from build123d import *

# Parameters (mm, degrees)
F1_DEPTH = 10
F2_DEPTH = 39
F3_R     = 1.27
F4_DEPTH = 39
F0_R     = 1.27
F5_DEPTH = 37


# Not quite as in the source:
# - a feature names something its author has since deleted; it is built from what else it names


with BuildPart() as f1:
    # F0 (on Top) → F1 (new body)
    with BuildSketch(Plane.XY):
        with BuildLine():
            Line((39.0916730868, 1.5), (-39.2084973779, 1.5))
            ThreePointArc((-39.2084973779, 1.5), (-39.0523737086, 0.7572105316), (-39, 0))
            ThreePointArc((-39, 0), (-39.0523737086, -0.7572105316), (-39.2084973779, -1.5))
            Line((-39.2084973779, -1.5), (35.8745669567, -1.5))
            Line((35.8745669567, -1.5), (39.0916730868, 1.5))
        make_face()
    extrude(amount=F1_DEPTH)

    # F0 (on Top) → F2 (join)
    with BuildSketch(Plane.XY):
        with BuildLine():
            ThreePointArc((-47.0597379557, -2.3869942602), (-46.8869942602, 2.5597379557), (-41.9402620443, 2.3869942602))
            Line((-41.9402620443, 2.3869942602), (-40.4775546411, 3.7509909803))
            ThreePointArc((-40.4775546411, 3.7509909803), (-48.2509909803, 4.0224453589), (-48.5224453589, -3.7509909803))
            Line((-48.5224453589, -3.7509909803), (-47.0597379557, -2.3869942602))
        make_face()
        with BuildLine():
            ThreePointArc((-41.9402620443, 2.3869942602), (-41.2435385121, 1.2827542935), (-41, 0))
            ThreePointArc((-41, 0), (-43.2172457065, -3.2564614879), (-47.0597379557, -2.3869942602))
            Line((-47.0597379557, -2.3869942602), (-48.5224453589, -3.7509909803))
            ThreePointArc((-48.5224453589, -3.7509909803), (-43.2079602627, -5.346085794), (-39.2084973779, -1.5))
            ThreePointArc((-39.2084973779, -1.5), (-39.0523737086, -0.7572105316), (-39, 0))
            ThreePointArc((-39, 0), (-39.0523737086, 0.7572105316), (-39.2084973779, 1.5))
            ThreePointArc((-39.2084973779, 1.5), (-39.7089513834, 2.7010836998), (-40.4775546411, 3.7509909803))
            Line((-40.4775546411, 3.7509909803), (-41.9402620443, 2.3869942602))
        make_face()
    extrude(amount=F2_DEPTH)

    # F3 (on face) → F4 (join)
    with BuildSketch(Plane.XY):
        with BuildLine():
            Line((-57.3884240397, 5.7566071407), (-48.5224453589, -3.7509909803))
            ThreePointArc((-48.5224453589, -3.7509909803), (-48.2509909803, 4.0224453589), (-40.4775546411, 3.7509909803))
            Line((-40.4775546411, 3.7509909803), (-49.3435333219, 13.2585891014))
            ThreePointArc((-49.3435333219, 13.2585891014), (-50.3882146293, 13.7346778018), (-51.4635614144, 13.3326221137))
            Line((-51.4635614144, 13.3326221137), (-57.3143910274, 7.8766352332))
            ThreePointArc((-57.3143910274, 7.8766352332), (-57.7904797278, 6.8319539259), (-57.3884240397, 5.7566071407))
        make_face()
        with Locations((-49.8572761974, 8.6775337363)):
            Circle(F3_R, mode=Mode.SUBTRACT)
    extrude(amount=F4_DEPTH)

    # F0 (on Top) → F5 (cut)
    with BuildSketch(Plane.XY):
        with BuildLine():
            ThreePointArc((-48.5224453589, -3.7509909803), (-48.2509909803, 4.0224453589), (-40.4775546411, 3.7509909803))
            Line((-40.4775546411, 3.7509909803), (-49.3435333219, 13.2585891014))
            ThreePointArc((-49.3435333219, 13.2585891014), (-50.3882146293, 13.7346778018), (-51.4635614144, 13.3326221137))
            Line((-51.4635614144, 13.3326221137), (-57.3143910274, 7.8766352332))
            ThreePointArc((-57.3143910274, 7.8766352332), (-57.7904797278, 6.8319539259), (-57.3884240397, 5.7566071407))
            Line((-57.3884240397, 5.7566071407), (-48.5224453589, -3.7509909803))
        make_face()
        with Locations((-49.8572761974, 8.6775337363)):
            Circle(F0_R, mode=Mode.SUBTRACT)
    extrude(amount=F5_DEPTH, mode=Mode.SUBTRACT)


solid = f1.part
Input: part model. Units: mm. Frame: model coordinates. A direction names the side the tool comes from. Give positions to 0.01 mm unless a question says otherwise; leave off trailing zeros. Order: outer loops, then holes, each group sorted by start corner. A loop starts at its lowest first (then second) coordinate and runs counter-clockwise, first axis right, second up. Notation, with made-up numbers: M -10,-38.75 L 1,-38.75 A22 cw 1,-26.75 Z; hole C -5.75,16 d4. An arc over 180 degrees is marked long. Answer as a JSON object with one key per item and string values.
1. Cut plane D-D, the plane y = 12. Output: boundary loops of the cut face in (x, z).
Result sheet:
{"outline": "M -52.89,37 L -48.17,37 L -48.17,39 L -52.89,39 Z"}
2. First-contact query: P1, Ø2, axis at x = -42, z = 20, coming from the +Y side; P2, Ø10, axis at y = -1, z = 16, coming from the -X side; P3, Ø3.5, axis at x = -16.5, y = 0.5, coming from the +Z side. Flat tips, straight axial feed; report the tip coordinate or a pass-through.
Result sheet:
{"P1": "y = 5.29", "P2": "x = -50", "P3": "z = 10"}
3. Cut plane A-A, the plane z = 8. Output: boundary loops of the cut face in (x, y).
Result sheet:
{"outline": "M -39.21,-1.5 L 35.87,-1.5 L 39.09,1.5 L -39.21,1.5 A5.5 ccw long Z; hole C -44.5,0 d7"}
4. Ray query, line 1 (Z direction, x = -52, y = 7); line 2 (Y direction, x = 16, z = 6); line 3 (Z direction, x = 20.5, y = -0.75). Return the intervals inside material, ascending. Write a range as [from, to].
Result sheet:
{"line 1": "[37, 39]", "line 2": "[-1.5, 1.5]", "line 3": "[0, 10]"}
5. Reachability of faces 1 (the flat face through (-1, 0, 10)), 2 (the flat face through (-2, -1.5, 5)), 3 (the flat face through (0, 1.5, 5)) from +Z, -Z, +X, -X, +Y, -Y: full face, straight path, thin tool, end or side. Return the list, or none.
Result sheet:
{"face 1": "+Z, +X, +Y, -Y", "face 2": "+Z, -Z, +X, -Y", "face 3": "+Z, -Z, +X, +Y"}
6. Cut plane C-C, the plane x = 26.5. Output: boundary loops of the cut face in (y, z), and give its area (3 significant figures).
Result sheet:
{"outline": "M -1.5,0 L 1.5,0 L 1.5,10 L -1.5,10 Z", "area": "30.0 mm²"}
7. Cut plane B-B, the plane x = -44.5. Output: boundary loops of the cut face in (y, z), and give its area (3 significant figures).
Result sheet:
{"outline": "M -5.5,0 L -3.5,0 L -3.5,39 L -5.5,39 Z; M 3.5,0 L 5.5,0 L 5.5,37 L 8.06,37 L 8.06,39 L 3.5,39 Z", "area": "161 mm²"}
8. Pull-direction query (Y, two-part tool) for faces 4 (the flat face through (37.46, -0.02, 4.93)), 5 (the cylindrical face through (-51.126, 8.733, 37.986)), 6 (the flat face through (-54.35, 10.64, 37.99)); classes: +Y half, -Y half, draft (parallel to the pull), parting line (faces both ways), or undercut.
Result sheet:
{"face 4": "-Y half", "face 5": "undercut", "face 6": "+Y half"}
